Input: part model. Units: mm. Frame: model coordinates. Give positions to 0.01 mm unless a question says otherwise; leave off trailing zeros. Write each loop counter-clockwise with the first axis right and the second up, starting at its lowest first coordinate (ties: lowest second). Pieces come first, ordered by that corner, then holes. Notation, with made-up numbers: (0, 45.5) -> (19, 45.5) arc R24 ccw to (19, 79.5) -> close; hole circle Ø1 at (71, 4). An arc over 180 degrees is marked (long way). Answer as a JSON object with one key per item and string values. Group by question number.
from build123d import *

# Parameters (mm, degrees)
EXTRUDE_1_DEPTH     = 3
SKETCH_2_R          = 2.6
SKETCH_2_R_2        = 1.6
SKETCH_2_R_3        = 6
CUT_EXTRUDE_1_DEPTH = 10


with BuildPart() as part:
    # 草图1 → 凸台-拉伸1 (new body)
    with BuildSketch(Plane.XY):
        Polygon((0, 0), (0, 40), (10, 40), (35, 65), (35, 110), (85, 110), (85, 65), (110, 40), (120, 40), (120, 0), align=None)
    extrude(amount=EXTRUDE_1_DEPTH)

    # 草图2 → 切除-拉伸1 (cut)
    with BuildSketch(Plane.XY.offset(3)):
        with Locations((45, 99)):
            Circle(SKETCH_2_R)
        with Locations((75, 99)):
            Circle(SKETCH_2_R)
        with Locations((75, 69)):
            Circle(SKETCH_2_R)
        with Locations((45, 69)):
            Circle(SKETCH_2_R)
        with Locations((8, 33)):
            Circle(SKETCH_2_R_2)
        with Locations((8, 7)):
            Circle(SKETCH_2_R_2)
        with Locations((112, 33)):
            Circle(SKETCH_2_R_2)
        with Locations((112, 7)):
            Circle(SKETCH_2_R_2)
        with Locations((20, 33)):
            Circle(SKETCH_2_R_2)
        with Locations((100, 33)):
            Circle(SKETCH_2_R_2)
        with Locations((20, 7)):
            Circle(SKETCH_2_R_2)
        with Locations((100, 7)):
            Circle(SKETCH_2_R_2)
        with Locations((32, 33)):
            Circle(SKETCH_2_R_2)
        with Locations((32, 7)):
            Circle(SKETCH_2_R_2)
        with Locations((88, 33)):
            Circle(SKETCH_2_R_2)
        with Locations((88, 7)):
            Circle(SKETCH_2_R_2)
        with Locations((60, 84)):
            Circle(SKETCH_2_R_3)
        with BuildLine():
            Line((43, 25), (77, 25))
            ThreePointArc((77, 25), (84, 18), (77, 11))
            Line((77, 11), (43, 11))
            ThreePointArc((43, 11), (36, 18), (43, 25))
        make_face()
    extrude(amount=-CUT_EXTRUDE_1_DEPTH, mode=Mode.SUBTRACT)


solid = part.part
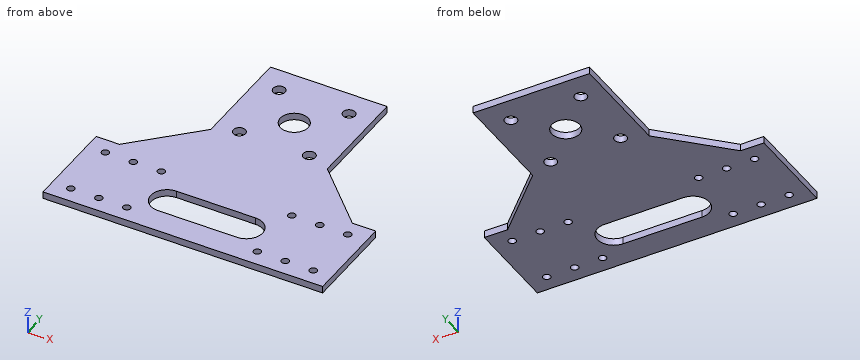
1. Section D-D (y = 33). Return the cut outline in (x, z).
2. Line query: line 1 (Y direction, x = 8, z = 2.15); line 2 (Y direction, x = 75, z = 1.55); line 3 (Y direction, x = 32, z = 1.95). Output: solid intervals per line, ascending.
3. Contact query for flat-ended pins moving along their axis: pin 1 Ø7 at (x, y) = (45, 99) entering from -Z; pin 2 Ø1.9 at (x, y) = (20, 7) entering from -Z; pin 3 Ø0.9 at (y, z) = (85, 1.5) entering from -X. Output: stop coordinate, or through.
4. Section C-C (z = 2.05). State how many separate pieces and enclosed holes the cut face has, plus the area to 3 significant figures.
5. Section A-A (x = 112). Return the cut outline in (y, z), plus the area to 3 significant figures.
6. Section B-B (y = 18). Return the cut outline in (x, z).
Working result:
{
 "1": {"outline": "(0, 0) -> (6.4, 0) -> (6.4, 3) -> (0, 3) -> close; (9.6, 0) -> (18.4, 0) -> (18.4, 3) -> (9.6, 3) -> close; (21.6, 0) -> (30.4, 0) -> (30.4, 3) -> (21.6, 3) -> close; (33.6, 0) -> (86.4, 0) -> (86.4, 3) -> (33.6, 3) -> close; (89.6, 0) -> (98.4, 0) -> (98.4, 3) -> (89.6, 3) -> close; (101.6, 0) -> (110.4, 0) -> (110.4, 3) -> (101.6, 3) -> close; (113.6, 0) -> (120, 0) -> (120, 3) -> (113.6, 3) -> close"},
 "2": {"line 1": "y = 0 to 5.4, 8.6 to 31.4, 34.6 to 40", "line 2": "y = 0 to 11, 25 to 66.4, 71.6 to 96.4, 101.6 to 110", "line 3": "y = 0 to 5.4, 8.6 to 31.4, 34.6 to 62"},
 "3": {"pin 1": "stops at z = 0", "pin 2": "passes through", "pin 3": "stops at x = 35"},
 "4": {"separate pieces": "1", "enclosed holes": "18", "area": "8,000 mm^2"},
 "5": {"outline": "(0, 0) -> (5.4, 0) -> (5.4, 3) -> (0, 3) -> close; (8.6, 0) -> (31.4, 0) -> (31.4, 3) -> (8.6, 3) -> close; (34.6, 0) -> (40, 0) -> (40, 3) -> (34.6, 3) -> close", "area": "101 mm^2"},
 "6": {"outline": "(0, 0) -> (36, 0) -> (36, 3) -> (0, 3) -> close; (84, 0) -> (120, 0) -> (120, 3) -> (84, 3) -> close"}
}
